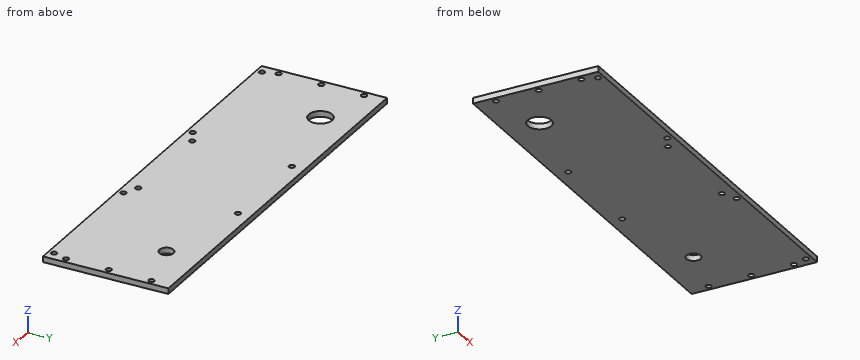
```python
from build123d import *

# Parameters (mm, degrees)
ESQUISSE1_W             = 284
ESQUISSE1_H             = 88
BOSS_EXTRU_1_DEPTH      = 4
ESQUISSE2_R             = 2
ESQUISSE2_R_2           = 8.25
ESQUISSE2_R_3           = 5
ENL_V_MAT_EXTRU_1_DEPTH = 298.348280641


with BuildPart() as part:
    # Esquisse1 → Boss.-Extru.1 (new body)
    with BuildSketch(Plane.XY):
        with Locations((142, 44)):
            Rectangle(ESQUISSE1_W, ESQUISSE1_H)
    extrude(amount=BOSS_EXTRU_1_DEPTH)

    # Esquisse2 → Enlèv. mat.-Extru.1 (cut, through all)
    with BuildSketch(Plane.XY.offset(4)):
        with Locations((107, 79)):
            Circle(ESQUISSE2_R)
        with Locations(Location((107, 9, 0), (0, 0, 180))):
            Circle(ESQUISSE2_R)
        with Locations((177, 9)):
            Circle(ESQUISSE2_R)
        with Locations(Location((177, 79, 0), (0, 0, 180))):
            Circle(ESQUISSE2_R)
        with Locations((42, 64)):
            Circle(ESQUISSE2_R_2)
        with Locations((4, 14)):
            Circle(ESQUISSE2_R)
        with Locations(Location((4, 74, 0), (0, 0, 180))):
            Circle(ESQUISSE2_R)
        with Locations((4, 44)):
            Circle(ESQUISSE2_R)
        with Locations(Location((280, 44, 0), (0, 0, 180))):
            Circle(ESQUISSE2_R)
        with Locations((280, 74)):
            Circle(ESQUISSE2_R)
        with Locations(Location((280, 14, 0), (0, 0, 180))):
            Circle(ESQUISSE2_R)
        with Locations((7, 4)):
            Circle(ESQUISSE2_R)
        with Locations((97, 4)):
            Circle(ESQUISSE2_R)
        with Locations(Location((187, 4, 0), (0, 0, 180))):
            Circle(ESQUISSE2_R)
        with Locations(Location((277, 4, 0), (0, 0, 180))):
            Circle(ESQUISSE2_R)
        with Locations((242, 64)):
            Circle(ESQUISSE2_R_3)
    extrude(amount=-ENL_V_MAT_EXTRU_1_DEPTH, mode=Mode.SUBTRACT)


solid = part.part
```
Input: part model. Units: mm. Frame: model coordinates. Give positions to 0.01 mm unless a question says otherwise; leave off trailing zeros. Order: outer loops, then holes, each group sorted by start corner. A loop starts at its lowest first (then second) coordinate and runs counter-clockwise, first axis right, second up. Notation, with made-up numbers: (81, -25) -> (134, -25) arc R12 cw to (134, -20) -> close; hole circle Ø1 at (54.5, 28). An arc over 180 degrees is marked (long way). Write each question's results on one line, items separated by ' | '. Start each with the question number.
Item 1: Contact query for a flat-ended pin moving along its axis: P1, Ø3, axis at x = 7, y = 4, coming from the -Z side. Output: stop coordinate, or through.
Item 2: Cut plane A-A on x = 242. Return the cut outline in (y, z).
Item 3: Cut plane B-B on z = 2.1. Give the number of separate pieces and of enclosed holes in the cut face, then the cut area to 3 significant figures.
Item 4: Line query: line 1 (X direction, y = 12.5, z = 3.3); line 2 (X direction, y = 80.5, z = 0.8); line 3 (X direction, y = 5, z = 1.2). Output: solid intervals per line, ascending.
Established:
1) P1: through
2) outline: (0, 0) -> (59, 0) -> (59, 4) -> (0, 4) -> close; (69, 0) -> (88, 0) -> (88, 4) -> (69, 4) -> close
3) separate pieces: 1 | enclosed holes: 16 | area: 24,500 mm^2
4) line 1: 0 to 2.68, 5.32 to 278.68, 281.32 to 284 | line 2: 0 to 105.68, 108.32 to 175.68, 178.32 to 284 | line 3: 0 to 5.27, 8.73 to 95.27, 98.73 to 185.27, 188.73 to 275.27, 278.73 to 284
